The drawing under review shows one solid part. Ordinate dimensions are in mm from its lowest x, y, z. A direction names the side the tool comes from. Give positions to 0.01 mm unless a question says otherwise; leave off trailing zeros. Order: outer loops, then holes, each group sorted by start corner. A loop starts at its lowest first (then second) coordinate and runs counter-clockwise, first axis right, second up. Notation, with made-up numbers: (34.25, 63.5) - (61.25, 63.5) arc R11 ccw to (61.25, 72.5) - close; hole circle Ø5 at (58.25, 25.5). An arc over 180 degrees is marked (long way). Answer as a JSON object with one key per item and string values. Group by question number.
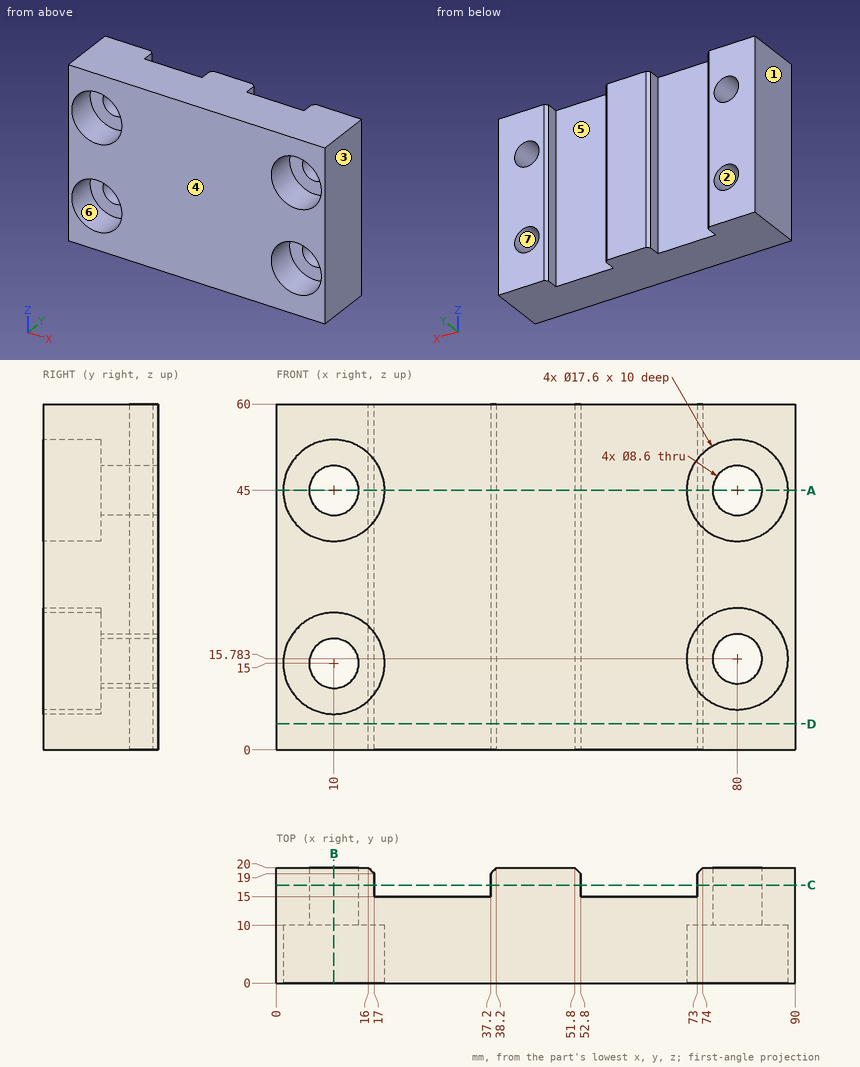
1) For the marked faces 5, 6 and 7, list the 3-axis set-ups (+Z, -Z, +X, -X, +Y, -Y) from which the entire face can be reached by the end or side of a thin tool; tool diameter is ignored.
2) Mouldability with a two-part tool opening along X and no side actions: class the marked faces 1, 2, 3 and 4 as released by +X, released by -X, zero draft, split by the parting line, or undercut.
3) Consider section C-C (y = 17). Give the boundary of the cut face in (x, z), plus the area to 3 significant figures.
4) Consider section D-D (z = 4.5). Give the boundary of the cut face in (x, y), plus the area to 3 significant figures.
5) For line 1 (Z direction, x = 80, y = 12.75); line 2 (Z direction, x = 10, y = 2.5); line 3 (X direction, y = 3.75, z = 17.5), list the stretches that pass through material, from the lowest coordinate up.
6) Consider section B-B (x = 10). Give the boundary of the cut face in (y, z), plus the area to 3 significant figures.
7) Consider section A-A (z = 45). Give the number of separate pieces and of enclosed holes in the cut face, plus the area to 3 significant figures.
8) For pin 1 (5.5 mm diameter, centred on x = 12.5, z = 17, fed in from -Y); pin 2 (6 mm diameter, centred on x = 29, z = 17, fed in from +Y), all flat-tipped, find the tip position at first contact; note any pin that passes through.
Result set:
{
 "1": {"face 5": "+Z, -Z, +Y", "face 6": "-Y", "face 7": "+Y, -Y"},
 "2": {"face 1": "released by -X", "face 2": "undercut", "face 3": "released by +X", "face 4": "zero draft"},
 "3": {"outline": "(0, 0) - (17, 0) - (17, 60) - (0, 60) - close; (37.2, 0) - (52.8, 0) - (52.8, 60) - (37.2, 60) - close; (73, 0) - (90, 0) - (90, 60) - (73, 60) - close; hole circle Ø8.6 at (10, 15); hole circle Ø8.6 at (10, 45); hole circle Ø8.6 at (80, 15.78); hole circle Ø8.6 at (80, 45)", "area": "2,740 mm2"},
 "4": {"outline": "(0, 0) - (90, 0) - (90, 20) - (74, 20) - (73, 19) - (73, 15) - (52.8, 15) - (52.8, 19) - (51.8, 20) - (38.2, 20) - (37.2, 19) - (37.2, 15) - (17, 15) - (17, 19) - (16, 20) - (0, 20) - close", "area": "1,600 mm2"},
 "5": {"line 1": "z = 0 to 11.48, 20.08 to 40.7, 49.3 to 60", "line 2": "z = 0 to 6.2, 23.8 to 36.2, 53.8 to 60", "line 3": "x = 0 to 1.56, 18.44 to 71.37, 88.63 to 90"},
 "6": {"outline": "(0, 0) - (20, 0) - (20, 10.7) - (10, 10.7) - (10, 6.2) - (0, 6.2) - close; (0, 23.8) - (10, 23.8) - (10, 19.3) - (20, 19.3) - (20, 40.7) - (10, 40.7) - (10, 36.2) - (0, 36.2) - close; (0, 53.8) - (10, 53.8) - (10, 49.3) - (20, 49.3) - (20, 60) - (0, 60) - close", "area": "676 mm2"},
 "7": {"separate pieces": "3", "enclosed holes": "0", "area": "1,070 mm2"},
 "8": {"pin 1": "stops at y = 10", "pin 2": "stops at y = 15"}
}
